```python
from build123d import *

# Parameters (mm, degrees)
SKETCH1_R           = 0.9
SKETCH1_R_2         = 1.05
BOSS_EXTRUDE2_DEPTH = 4


with BuildPart() as part:
    # Sketch1 → Boss-Extrude2 (new body)
    with BuildSketch(Plane(origin=(0, 0, 0), x_dir=(1, 0, 0), z_dir=(0, 1, 0))):
        with BuildLine():
            Line((0, 51.3), (0, 53))
            add(Edge.make_bspline(
                [(0, 53), (-11.288586004, 48.107069446), (-18.25, 38.69126661), (-18.25, 23.6)],
                knots=[0, 0, 0, 0, 1, 1, 1, 1], degree=3))
            Line((-18.25, 23.6), (-18.25, 22))
            ThreePointArc((-18.25, 22), (-17.078427125, 19.171572875), (-14.25, 18))
            Line((-14.25, 18), (-2.8, 18))
            ThreePointArc((-2.8, 18), (-0.6, 20.2), (-2.8, 22.4))
            ThreePointArc((-2.8, 22.4), (-9.397521131, 27.257683793), (-6.717797887, 35))
            ThreePointArc((-6.717797887, 35), (-6.044737279, 42.503576591), (0, 47))
            Line((0, 47), (0, 48.7))
            ThreePointArc((0, 48.7), (-1.3, 50), (0, 51.3))
        make_face()
        with Locations(Location((-2.8, 20.2, 0), (0, 0, 270))):
            Circle(SKETCH1_R, mode=Mode.SUBTRACT)
        with Locations(Location((-14.25, 22, 0), (0, 0, 270))):
            Circle(SKETCH1_R_2, mode=Mode.SUBTRACT)
    extrude(amount=BOSS_EXTRUDE2_DEPTH)


solid = part.part
```
Design review of the part built by this model. Coordinates are the model's own, in mm. Coordinates: 2 decimals unless noted, no trailing zeros. Write each loop counter-clockwise with the first axis right and the second up, starting at its lowest first coordinate (ties: lowest second). Pieces come first, ordered by that corner, then holes. Notation, with made-up numbers: M -30.5,-26 L 27.5,-26 A10 ccw 27.5,-8 Z; hole C -23,25 d10. An arc over 180 degrees is marked long. Answer as a JSON object with one key per item and string values.
Item 1: Add section A-A, the plane z = -20.2. Give the boundary of the cut face in (x, y).
Outcome:
{"outline": "M -17.82,0 L -3.7,0 L -3.7,4 L -17.82,4 Z; M -1.9,0 L -0.6,0 L -0.6,4 L -1.9,4 Z"}
Item 2: Wall thickness on probe 1 along Z at (x, y) = (-3, 2.85); probe 2 along Z at (x, y) = (-1, 1.45); probe 3 along X at (y, z) = (2.4, -22): over which ranges is each line inside the solid? List them lowest first.
Outcome:
{"probe 1": "-51.54 to -45.75, -22.4 to -21.08, -19.32 to -18", "probe 2": "-52.55 to -50.83, -49.17 to -46.72, -21.46 to -18.94", "probe 3": "-18.25 to -15.3, -13.2 to -1.54"}
Item 3: Add section B-B, the plane y = 1.4. State how many separate pieces and enclosed holes the cut face has, and give its area (3 significant figures).
Outcome:
{"separate pieces": "1", "enclosed holes": "2", "area": "307 mm²"}
Item 4: Draft analysis for pull direction X (two halves, no side actions). For faces 1 (the flat face through (0, 2, -48)), 2 (the cylindrical face through (-13.21, 1.97, -22.14)), 3 (the flat face through (-9, 2, -18)), state which applies: pulls with the +X half, pulls with the -X half, needs draft (parallel to the pull), parting line crosses it, or undercut.
Outcome:
{"face 1": "pulls with the +X half", "face 2": "undercut", "face 3": "needs draft"}
